Geometry check sheet. Reference: the model listing, model coordinates, mm. A direction names the side the tool comes from. Coordinates: 2 decimals unless noted, no trailing zeros. Order: outer loops, then holes, each group sorted by start corner. A loop starts at its lowest first (then second) coordinate and runs counter-clockwise, first axis right, second up. Notation, with made-up numbers: M 28.25,-28.5 L 63.25,-28.5 A27 cw 63.25,-6.5 Z; hole C 77.5,63.5 d10. An arc over 180 degrees is marked long. One line per item, written item: value. Start each with the question number.
1) Sectioned sample at C-C, the plane z = 4. Enter the section's corners in (x, y) (3 decimals).
2) Sectioned sample at A-A, the plane y = 22. Enter the section's corners in (x, z), then the cut area to 3 significant figures.
3) Sectioned sample at B-B, the plane x = 33. Enter the section's corners in (y, z) (3 decimals).
4) Thickness scan on L1, parallel to Z at x = 35.25, y = 14.5; L2, parallel to Y at x = 31.5, z = -11 (3 decimals); L3, parallel to X at y = 21.5, z = 38. Record the ranges inside material, lowest first. Write a range as from..to.
5) Access from +Z, -Z, +X, -X, +Y, -Y to the whole of each face (thin tool, end or side, straight path). Record for faces 1 (the flat face through (29.4, 14, -29)), 2 (the flat face through (33, 15.875, 4)), 3 (the flat face through (21.463, 22, 4)).
6) Sectioned sample at D-D, the plane y = 14.5. State how many separate pieces and enclosed holes the cut face has, then the cut area to 3 significant figures.
7) Go/stop test with a flat-tipped pin: P1, Ø6.5, axis at y = 20.88, z = 26.72, coming from the +X side. Record where the tip stops, or that it passes through.
8) Draft check along Z on faces 4 (the flat face through (24, 19, 53.947)), 5 (the flat face through (35.75, 14, 35)), 6 (the flat face through (31, 12.7, 4)). Enter one of: pulls with the +Z half, pulls with the -Z half, needs draft (parallel to the pull), parting line crosses it, or undercut.
```python
from build123d import *

# Parameters (mm, degrees)
EXTRUDE1_DEPTH     = 50.8
CUT_EXTRUDE1_DEPTH = 70.3077329
SKETCH4_R          = 2.54
CUT_EXTRUDE2_DEPTH = 65.578023899


with BuildPart() as part:
    # Sketch1 → Extrude1 (new, symmetric)
    with BuildSketch(Plane.XY.offset(3.146668532)):
        Polygon((21.463, 31.75), (21.463, 12.7), (40.513, 12.7), (40.513, 15.875), (24.638, 15.875), (24.638, 31.75), align=None)
    extrude(amount=EXTRUDE1_DEPTH, both=True)

    # Sketch3 → Cut-Extrude1 (cut, through all)
    with BuildSketch(Plane(origin=(0, 15.875, 0), x_dir=(-1, 0, 0), z_dir=(0, 1, 0))):
        with BuildLine():
            Line((-35.7505, -34.953331468), (-35.7505, -22.253331468))
            ThreePointArc((-35.7505, -22.253331468), (-32.5755, -19.078331468), (-29.4005, -22.253331468))
            Line((-29.4005, -22.253331468), (-29.4005, -34.953331468))
            ThreePointArc((-29.4005, -34.953331468), (-32.5755, -38.128331468), (-35.7505, -34.953331468))
        make_face()
        with BuildLine():
            Line((-29.4005, 41.246668532), (-29.4005, 28.546668532))
            ThreePointArc((-29.4005, 28.546668532), (-32.5755, 25.371668532), (-35.7505, 28.546668532))
            Line((-35.7505, 28.546668532), (-35.7505, 41.246668532))
            ThreePointArc((-35.7505, 41.246668532), (-32.5755, 44.421668532), (-29.4005, 41.246668532))
        make_face()
    extrude(amount=-CUT_EXTRUDE1_DEPTH, mode=Mode.SUBTRACT)

    # Sketch4 → Cut-Extrude2 (cut, through all)
    with BuildSketch(Plane(origin=(24.638, 0, 0), x_dir=(0, 0, -1), z_dir=(1, 0, 0))):
        with Locations((20.424531468, 20.8788)):
            Circle(SKETCH4_R)
        with Locations((-26.717868532, 20.8788)):
            Circle(SKETCH4_R)
    extrude(amount=-CUT_EXTRUDE2_DEPTH, mode=Mode.SUBTRACT)


solid = part.part
```
Final values:
1. outline: M 21.463,12.7 L 40.513,12.7 L 40.513,15.875 L 24.638,15.875 L 24.638,31.75 L 21.463,31.75 Z
2. outline: M 21.46,-47.65 L 24.64,-47.65 L 24.64,-22.7 L 21.46,-22.7 Z; M 21.46,-18.15 L 24.64,-18.15 L 24.64,24.44 L 21.46,24.44 Z; M 21.46,29 L 24.64,29 L 24.64,53.95 L 21.46,53.95 Z
2. area: 294 mm^2
3. outline: M 12.7,-47.653 L 15.875,-47.653 L 15.875,-38.1 L 12.7,-38.1 Z; M 12.7,-19.107 L 15.875,-19.107 L 15.875,25.4 L 12.7,25.4 Z; M 12.7,44.393 L 15.875,44.393 L 15.875,53.947 L 12.7,53.947 Z
4. L1: z = -47.65..-36.66, -20.54..26.84, 42.96..53.95
4. L2: y = 12.7..15.875
4. L3: x = 21.46..24.64
5. face 1: +Y, -Y
5. face 2: +Z, -Z, +X, +Y
5. face 3: +Z, -Z, -X, +Y, -Y
6. separate pieces: 1
6. enclosed holes: 2
6. area: 1,710 mm^2
7. P1: stops at x = 24.64
8. face 4: pulls with the +Z half
8. face 5: undercut
8. face 6: needs draft
